Job drawing, mm, ordinate dimensions from the low corner. One solid piece. A direction names the side the tool comes from. Round coordinates to 2 decimals unless told otherwise and drop trailing zeros. Loops run counter-clockwise (first coordinate to the right, second up) from the corner with the lowest first, then second, coordinate; pieces in that order, holes last. Notation, with made-up numbers: M 81.5,-13.75 L 87.5,-13.75 A6 cw 87.5,-7.75 Z; hole C 80.25,42 d8. An arc over 180 degrees is marked long. Use a Markdown table: item, result. Add a question column.
(1) Band-saw the part on D-D, the plane z = 14.25. Write the cut outline in (x, y) (1 decimal).
(2) Band-saw the part on C-C, the plane y = 80. Write the cut outline in (x, z).
(3) Band-saw the part on B-B, the plane x = 65. Write the cut outline in (y, z).
(4) Wall check: L1, parallel to Y at x = 42.7, z = 9 (1 decimal); L2, parallel to Y at x = 39, z = 8.75 (1 decimal); L3, parallel to X at y = 71.5, z = 8 (1 decimal). Give the ranges that are in metal, low to high.
(5) Which spindle directions (+Z, -Z, +X, -X, +Y, -Y) get a long thin tool onto all of the face, cutting with end or side? Do the marked faces 1, 2 and 3. Say none if no direction does.
(6) Two-plate mould, pull along X, no slides. Class the marked faces 4, 5, 6 and 7: released by +X, released by -X, zero draft, split by the parting line, or undercut.
(7) Flat gauge pins, fed straight in: P1, Ø3, axis at x = 32.5, y = 73.5, coming from the +Z side; P2, Ø5, axis at x = 67, z = 11.5, coming from the +Y side; P3, Ø1, axis at y = 62.5, z = 7, coming from the +X side (1 decimal); P4, Ø8, axis at y = 67.5, z = 10.5, coming from the +X side. Where does each tip first touch, or does it go through?
(8) Band-saw the part on A-A, the plane x = 42.7. Write the cut outline in (y, z) (1 decimal).
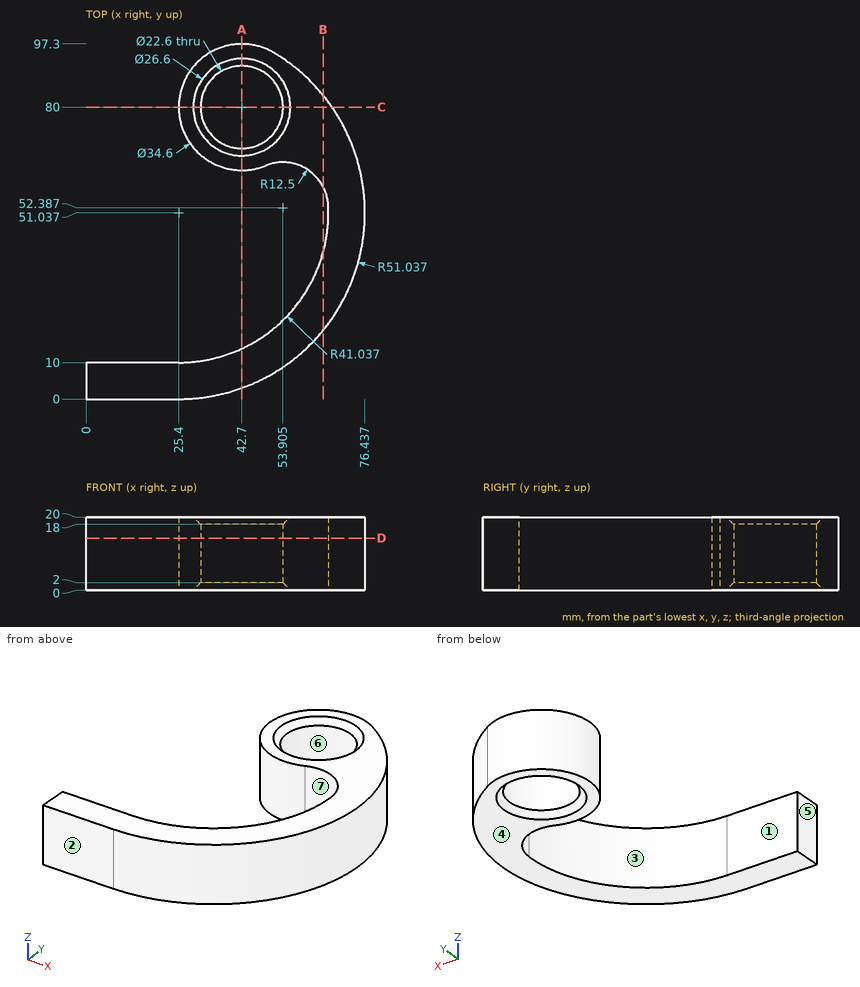
Return value:
| question | item | result |
|---|---|---|
| 1 | outline | M 0,0 L 25.4,0 A51 ccw 51.6,94.9 A17.3 ccw long 49.2,64 A12.5 cw 66.4,53 A41 cw 25.4,10 L 0,10 Z; hole C 42.7,80 d22.6 |
| 2 | outline | M 25.4,0 L 29.4,0 L 31.4,2 L 31.4,18 L 29.4,20 L 25.4,20 Z; M 54,2 L 56,0 L 67.42,0 L 67.42,20 L 56,20 L 54,18 Z |
| 3 | outline | M 18.84,0 L 40.27,0 L 40.27,20 L 18.84,20 Z; M 58.14,0 L 83.23,0 L 83.23,20 L 58.14,20 Z |
| 4 | L1 | 3 to 13.8, 62.7 to 68.7, 91.3 to 97.3 |
| 4 | L2 | 1.8 to 12.3, 63.1 to 69.3, 90.7 to 96.9 |
| 4 | L3 | 27.6 to 35.3, 50.1 to 72.2 |
| 5 | face 1 | +Z, -Z, -X, +Y |
| 5 | face 2 | +Z, -Z, +X, -X, -Y |
| 5 | face 3 | +Z, -Z, -X |
| 6 | face 4 | zero draft |
| 6 | face 5 | released by -X |
| 6 | face 6 | undercut |
| 6 | face 7 | undercut |
| 7 | P1 | z = 20 |
| 7 | P2 | y = 83.84 |
| 7 | P3 | x = 75.2 |
| 7 | P4 | x = 74.89 |
| 8 | outline | M 3,0 L 13.8,0 L 13.8,20 L 3,20 Z; M 62.7,0 L 66.7,0 L 68.7,2 L 68.7,18 L 66.7,20 L 62.7,20 Z; M 91.3,2 L 93.3,0 L 97.3,0 L 97.3,20 L 93.3,20 L 91.3,18 Z |
